Geometry: final body of the model. Coordinates: model frame, mm. A direction names the side the tool comes from. Give positions to 0.01 mm unless a question says otherwise; leave off trailing zeros. Order: outer loops, then holes, each group sorted by start corner. A loop starts at its lowest first (then second) coordinate and runs counter-clockwise, first axis right, second up. Notation, with made-up numbers: (39.5, 66) - (43.5, 66) arc R6 cw to (43.5, 72) - close; hole circle Ø1 at (44.25, 44). An arc over 180 degrees is marked (long way). One line per question, with ' | ' between items. Start each with the question number.
from build123d import *

# Parameters (mm, degrees)
SKETCH1_W                            = 15.24
SKETCH1_H                            = 2.54
BASE_EXTRUDE_DEPTH                   = 1.27
PIN_DEPTH                            = 0.3175
PIN_CHAMFER_SIZE2                    = 0.184896879
PIN_CHAMFER_SIZE                     = 0.508
PIN_PATTERN_COUNT                    = 3
PIN_PATTERN_PITCH                    = 5.08
PIN_CHAMFER_OF_PIN_PATTERN_SIZE2     = 0.184896879
PIN_CHAMFER_OF_PIN_PATTERN_SIZE      = 0.508
PIN_2_DEPTH                          = 0.3175
PIN_2_CHAMFER_SIZE2                  = 0.184896879
PIN_2_CHAMFER_SIZE                   = 0.508
PIN_2_PATTERN_COUNT                  = 3
PIN_2_PATTERN_PITCH                  = 5.08
PIN_2_CHAMFER_OF_PIN_2_PATTERN_SIZE2 = 0.184896879
PIN_2_CHAMFER_OF_PIN_2_PATTERN_SIZE  = 0.508
SV_CUT_DEPTH                         = 4.5
SV_CUT_PATTERN_COUNT                 = 5
SV_CUT_PATTERN_PITCH                 = 2.54
LPATTERN1_COUNT                      = 3
LPATTERN1_PITCH                      = 2.54
SKETCH16_W                           = 7.62
SKETCH16_H                           = 5.30254
CUT_EXTRUDE1_DEPTH                   = 9


with BuildPart() as part:
    # Sketch1 → Base Extrude (new body, symmetric)
    with BuildSketch(Plane(origin=(0, 0, 0), x_dir=(1, 0, 0), z_dir=(0, 1, 0))):
        with Locations((6.35, 0)):
            Rectangle(SKETCH1_W, SKETCH1_H)
    extrude(amount=BASE_EXTRUDE_DEPTH, both=True)

    # Sketch8 → Pin (add, symmetric)
    with BuildSketch(Plane(origin=(0, 0, 0), x_dir=(0, 0, -1), z_dir=(1, 0, 0))):
        with BuildLine():
            Line((0.32004, -1.087), (0.32004, 5.262))
            Line((0.32004, 5.262), (0.135143121, 5.77))
            Line((0.135143121, 5.77), (-0.130063121, 5.77))
            Line((-0.130063121, 5.77), (-0.31496, 5.262))
            Line((-0.31496, 5.262), (-0.31496, -1.214))
            ThreePointArc((-0.31496, -1.214), (-0.01738049, -1.93242049), (0.70104, -2.23))
            Line((0.70104, -2.23), (2.142, -2.23))
            Line((2.142, -2.23), (2.65, -2.045103121))
            Line((2.65, -2.045103121), (2.65, -1.779896879))
            Line((2.65, -1.779896879), (2.142, -1.595))
            Line((2.142, -1.595), (0.82804, -1.595))
            ThreePointArc((0.82804, -1.595), (0.468829755, -1.446210245), (0.32004, -1.087))
        make_face()
    pin = extrude(amount=PIN_DEPTH, both=True)

    # Pin Chamfer
    pin_chamfer_edges = [part.edges().sort_by_distance(p)[0] for p in [
        (0.3175, -1.9125, -2.65),
        (-0.3175, 5.77, -0.00254),
        (-0.3175, -1.9125, -2.65),
        (0.3175, 5.77, -0.00254),
    ]]
    chamfer(pin_chamfer_edges, length=PIN_CHAMFER_SIZE, length2=PIN_CHAMFER_SIZE2)

    # Pin Pattern: Pin ×3
    with Locations(*[(i * PIN_PATTERN_PITCH, 0, 0) for i in range(1, PIN_PATTERN_COUNT)]):
        add(pin)

    # Pin Chamfer of Pin Pattern
    pin_chamfer_of_pin_pattern_edges = [part.edges().sort_by_distance(p)[0] for p in [
        (5.3975, -1.9125, -2.65),
        (4.7625, 5.77, -0.00254),
        (4.7625, -1.9125, -2.65),
        (5.3975, 5.77, -0.00254),
        (10.4775, -1.9125, -2.65),
        (9.8425, 5.77, -0.00254),
        (9.8425, -1.9125, -2.65),
        (10.4775, 5.77, -0.00254),
    ]]
    chamfer(pin_chamfer_of_pin_pattern_edges, length=PIN_CHAMFER_OF_PIN_PATTERN_SIZE, length2=PIN_CHAMFER_OF_PIN_PATTERN_SIZE2)

    # Sketch9 → Pin 2 (add, symmetric)
    with BuildSketch(Plane(origin=(2.54, 0, 0), x_dir=(0, 0, -1), z_dir=(1, 0, 0))):
        with BuildLine():
            Line((-0.32004, -1.087), (-0.32004, 5.262))
            Line((-0.32004, 5.262), (-0.135143121, 5.77))
            Line((-0.135143121, 5.77), (0.130063121, 5.77))
            Line((0.130063121, 5.77), (0.31496, 5.262))
            Line((0.31496, 5.262), (0.31496, -1.214))
            ThreePointArc((0.31496, -1.214), (0.01738049, -1.93242049), (-0.70104, -2.23))
            Line((-0.70104, -2.23), (-2.14454, -2.23))
            Line((-2.14454, -2.23), (-2.65254, -2.045103121))
            Line((-2.65254, -2.045103121), (-2.65254, -1.779896879))
            Line((-2.65254, -1.779896879), (-2.14454, -1.595))
            Line((-2.14454, -1.595), (-0.82804, -1.595))
            ThreePointArc((-0.82804, -1.595), (-0.468829755, -1.446210245), (-0.32004, -1.087))
        make_face()
    pin_2 = extrude(amount=PIN_2_DEPTH, both=True)

    # Pin 2 Chamfer
    pin_2_chamfer_edges = [part.edges().sort_by_distance(p)[0] for p in [
        (2.8575, -1.9125, 2.65254),
        (2.2225, -1.9125, 2.65254),
        (2.2225, 5.77, 0.00254),
        (2.8575, 5.77, 0.00254),
    ]]
    chamfer(pin_2_chamfer_edges, length=PIN_2_CHAMFER_SIZE, length2=PIN_2_CHAMFER_SIZE2)

    # Pin 2 Pattern: Pin 2 ×3
    with Locations(*[(i * PIN_2_PATTERN_PITCH, 0, 0) for i in range(1, PIN_2_PATTERN_COUNT)]):
        add(pin_2)

    # Pin 2 Chamfer of Pin 2 Pattern
    pin_2_chamfer_of_pin_2_pattern_edges = [part.edges().sort_by_distance(p)[0] for p in [
        (7.9375, -1.9125, 2.65254),
        (7.3025, -1.9125, 2.65254),
        (7.3025, 5.77, 0.00254),
        (7.9375, 5.77, 0.00254),
        (13.0175, -1.9125, 2.65254),
        (12.3825, -1.9125, 2.65254),
        (12.3825, 5.77, 0.00254),
        (13.0175, 5.77, 0.00254),
    ]]
    chamfer(pin_2_chamfer_of_pin_2_pattern_edges, length=PIN_2_CHAMFER_OF_PIN_2_PATTERN_SIZE, length2=PIN_2_CHAMFER_OF_PIN_2_PATTERN_SIZE2)

    # Sketch15 → SV Cut (cut, through all)
    with BuildSketch(Plane(origin=(0, 1.27, 0), x_dir=(-1, 0, 0), z_dir=(0, 1, 0))):
        Polygon((-3.556, 1.27), (-3.702646976, 1.016), (-3.917353024, 1.016), (-4.064, 1.27), align=None)
        Polygon((-4.064, -1.27), (-3.917353024, -1.016), (-3.702646976, -1.016), (-3.556, -1.27), align=None)
    sv_cut = extrude(amount=-SV_CUT_DEPTH, mode=Mode.SUBTRACT)

    # SV Cut Pattern: SV Cut ×5
    with Locations(*[(i * SV_CUT_PATTERN_PITCH, 0, 0) for i in range(1, SV_CUT_PATTERN_COUNT)]):
        add(sv_cut, mode=Mode.SUBTRACT)

    # LPattern1: SV Cut ×3
    with Locations(*[(-i * LPATTERN1_PITCH, 0, 0) for i in range(1, LPATTERN1_COUNT)]):
        add(sv_cut, mode=Mode.SUBTRACT)

    # Sketch16 → Cut-Extrude1 (cut, through all)
    with BuildSketch(Plane(origin=(0, 5.77, 0), x_dir=(1, 0, 0), z_dir=(0, 1, 0))):
        with Locations((10.16, -0.00127)):
            Rectangle(SKETCH16_W, SKETCH16_H)
    extrude(amount=-CUT_EXTRUDE1_DEPTH, mode=Mode.SUBTRACT)


solid = part.part
(1) Access query for faces 5 (the flat face through (0.318, -2, -1)), 6 (the flat face through (3, 0, 1.27)), 7 (the cylindrical face through (5.08, -1.94, 0.01)), 8 (the flat face through (0, 0, -1.27)), 9 (the cylindrical face through (2.54, -1.94, -0.01)). Directions: +Z, -Z, +X, -X, +Y, -Y. A direction counts if a zero-diameter tool reaches every point of the face in a straight line with its end or side. Return the directions, or none.
(2) Cut plane D-D, the plane x = 4.5. Return the cut outline in (y, z).
(3) Cut plane A-A, the plane y = 2.5. Return the cut outline in (x, z), plus the area to 3 significant figures.
(4) Cut plane C-C, the plane y = -0.5. Return the cut outline in (x, z), plus the area to 3 significant figures.
(5) Cut plane B-B, the plane z = -1.6. Return the cut outline in (x, y) (1 decimal), plus the area to 3 significant figures.
(6) Contact query for flat-ended pins moving along their axis: P1, Ø1, axis at x = 0.5, y = -0.5, coming from the -Z side; P2, Ø0.7, axis at x = 2.5, z = 1.5, coming from the +Y side; P3, Ø0.5, axis at y = -2, z = -0.5, coming from the -X side. Output: stop coordinate, or through.
(7) Material intervals for line 1 along X through (y, z) = (2, 0); line 2 along Y through (x, z) = (1.75, 0); line 3 along Z through (x, y) = (5.25, 3.25), sorted ascending. Write a range as from..to.
(8) Pull-direction query (X, two-part tool) for faces 1 (the flat face through (-0.318, -2, -1)), 2 (the flat face through (0, 0, 1.27)), 3 (the flat face through (2.858, -2, 1)), 4 (the flat face through (5.398, -2, -1)); classes: +X half, -X half, draft (parallel to the pull), parting line (faces both ways), or undercut.
Results are:
1) face 5: +Z, -Z, -Y | face 6: +Z, +X, -X, +Y | face 7: +Z, +X, -Y | face 8: -Z, +X, -X, +Y | face 9: -Z, -Y
2) outline: (-1.27, -1.27) - (1.27, -1.27) - (1.27, 1.27) - (-1.27, 1.27) - close
3) outline: (-0.32, -0.32) - (0.32, -0.32) - (0.32, 0.31) - (-0.32, 0.31) - close; (2.22, -0.31) - (2.86, -0.31) - (2.86, 0.32) - (2.22, 0.32) - close; (4.76, -0.32) - (5.4, -0.32) - (5.4, 0.31) - (4.76, 0.31) - close | area: 1.21 mm2
4) outline: (-1.27, -1.02) - (-1.16, -1.02) - (-1.02, -1.27) - (1.02, -1.27) - (1.16, -1.02) - (1.38, -1.02) - (1.52, -1.27) - (3.56, -1.27) - (3.7, -1.02) - (3.92, -1.02) - (4.06, -1.27) - (6.1, -1.27) - (6.24, -1.02) - (6.35, -1.02) - (6.35, 1.02) - (6.24, 1.02) - (6.1, 1.27) - (4.06, 1.27) - (3.92, 1.02) - (3.7, 1.02) - (3.56, 1.27) - (1.52, 1.27) - (1.38, 1.02) - (1.16, 1.02) - (1.02, 1.27) - (-1.02, 1.27) - (-1.16, 1.02) - (-1.27, 1.02) - close | area: 18.8 mm2
5) outline: (-0.3, -2.2) - (0.3, -2.2) - (0.3, -1.6) - (-0.3, -1.6) - close; (4.8, -2.2) - (5.4, -2.2) - (5.4, -1.6) - (4.8, -1.6) - close | area: 0.806 mm2
6) P1: z = -1.27 | P2: y = 1.27 | P3: x = -0.32
7) line 1: -0.32..0.32, 2.22..2.86, 4.76..5.4 | line 2: -1.27..1.27 | line 3: -0.32..0.31
8) face 1: -X half | face 2: draft | face 3: undercut | face 4: +X half
